Source: CAD feature listing. Evaluate the final solid. Frame: model axes, mm. A direction names the side the tool comes from. Give positions to 0.01 mm unless a question says otherwise; leave off trailing zeros. Loops run counter-clockwise (first coordinate to the right, second up) from the corner with the lowest first, then second, coordinate; pieces in that order, holes last. Notation, with made-up numbers: (49.25, 52) -> (84.25, 52) arc R31 ccw to (84.25, 78) -> close; hole circle Ø6 at (47.5, -35.5). An arc over 180 degrees is marked (long way). Put each result on its own line as item: value.
```python
from build123d import *

# Parameters (mm, degrees)
BOSS_EXTRU_2_DEPTH = 40


with BuildPart() as part:
    # Esquisse1 → Boss.-Extru.2 (new body)
    with BuildSketch(Plane.XY):
        Polygon((-132.286889429, -48.932516673), (-154.786889429, -31.932516673), (-154.786889429, -46.932516673), (-159.786889429, -46.932516673), (-159.786889429, -31.932516673), (-182.286889429, -48.932516673), align=None)
        Polygon((-138.251616171, -46.932516673), (-152.786889429, -35.950310211), (-152.786889429, -46.932516673), align=None, mode=Mode.SUBTRACT)
        Polygon((-176.322162687, -46.932516673), (-161.786889429, -35.950310211), (-161.786889429, -46.932516673), align=None, mode=Mode.SUBTRACT)
    extrude(amount=BOSS_EXTRU_2_DEPTH)


solid = part.part
```
(1) Reachability of faces 1 (the flat face through (-154, -43, 0)), 2 (the flat face through (-146, -46.933, 20)), 3 (the flat face through (-159.787, -40, 20)) from +Z, -Z, +X, -X, +Y, -Y: full face, straight path, thin tool, end or side. Return the list, or none.
Calculated:
face 1: -Z, +X, -X, +Y, -Y
face 2: +Z, -Z
face 3: +Z, -Z, +Y
(2) Section A-A on z = 26. Return loops of the section in (x, y), then the cut area to 3 significant figures.
Calculated:
outline: (-182.29, -48.93) -> (-132.29, -48.93) -> (-154.79, -31.93) -> (-154.79, -46.93) -> (-159.79, -46.93) -> (-159.79, -31.93) -> close; hole (-176.32, -46.93) -> (-161.79, -46.93) -> (-161.79, -35.95) -> close; hole (-152.79, -46.93) -> (-138.25, -46.93) -> (-152.79, -35.95) -> close
area: 233 mm²
(3) Section C-C on y = -34. Return loops of the section in (x, z).
Calculated:
outline: (-162.52, 0) -> (-159.79, 0) -> (-159.79, 40) -> (-162.52, 40) -> close; (-154.79, 0) -> (-152.05, 0) -> (-152.05, 40) -> (-154.79, 40) -> close
(4) First-contact query: P1, Ø1, axis at y = -39.5, z = 5.5, coming from the +X side; P2, Ø8, axis at x = -143.5, z = 29, coming from the +Y side; P3, Ø2, axis at x = -138.5, z = 29, coming from the +Y side. Flat tips, straight axial feed; report the tip coordinate or a pass-through.
Calculated:
P1: stops at x = -144.11
P2: stops at y = -37.44
P3: stops at y = -43.48
(5) Line query: probe 1 along X at (y, z) = (-46.5, 30); probe 2 along X at (y, z) = (-38.5, 9); probe 3 along X at (y, z) = (-33.5, 30). Output: solid intervals per line, ascending. Write a range as from..to.
Calculated:
probe 1: x = -179.07..-175.75, -161.79..-159.79, -154.79..-152.79, -138.82..-135.51
probe 2: x = -168.48..-165.16, -161.79..-159.79, -154.79..-152.79, -149.41..-146.09
probe 3: x = -161.86..-159.79, -154.79..-152.71
(6) Draft query along X for faces 4 (the flat face through (-161.787, -41, 20)), 5 (the flat face through (-158, -48.933, 20)), 6 (the flat face through (-157, -46.933, 20)), 7 (the flat face through (-170.879, -40.314, 19.72)). Return one class per face: released by +X, released by -X, zero draft, split by the parting line, or undercut.
Calculated:
face 4: undercut
face 5: zero draft
face 6: undercut
face 7: released by -X
(7) Section B-B on x = -148. Return loops of the section in (y, z), then the cut area to 3 significant figures.
Calculated:
outline: (-48.93, 0) -> (-46.93, 0) -> (-46.93, 40) -> (-48.93, 40) -> close; (-39.57, 0) -> (-37.06, 0) -> (-37.06, 40) -> (-39.57, 40) -> close
area: 180 mm²
(8) Section D-D on y = -41. Return loops of the section in (x, z).
Calculated:
outline: (-171.79, 0) -> (-168.47, 0) -> (-168.47, 40) -> (-171.79, 40) -> close; (-161.79, 0) -> (-159.79, 0) -> (-159.79, 40) -> (-161.79, 40) -> close; (-154.79, 0) -> (-152.79, 0) -> (-152.79, 40) -> (-154.79, 40) -> close; (-146.1, 0) -> (-142.79, 0) -> (-142.79, 40) -> (-146.1, 40) -> close
